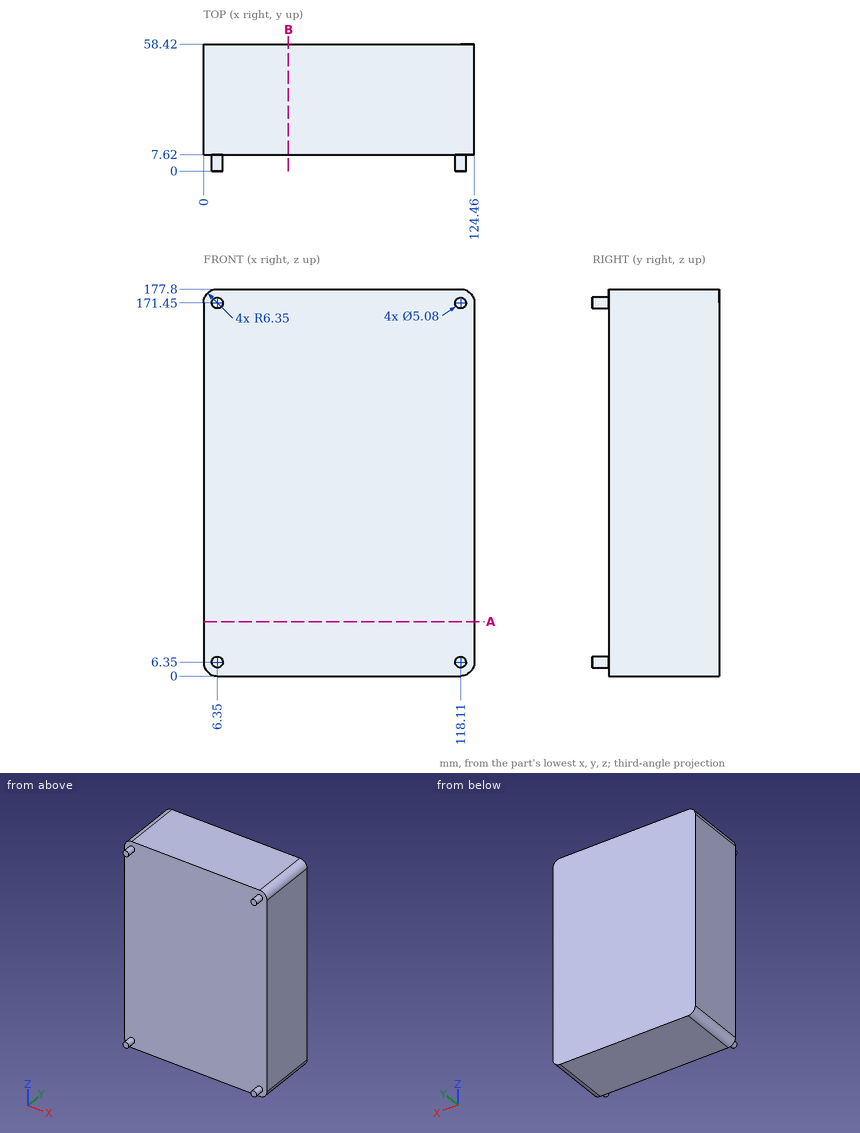
Geometry check sheet. Reference: drawing and pictorial views, mm from the part's lowest x, y, z. Give positions to 0.01 mm unless a question says otherwise; leave off trailing zeros. Order: outer loops, then holes, each group sorted by start corner. A loop starts at its lowest first (then second) coordinate and runs counter-clockwise, first axis right, second up. Notation, with made-up numbers: (81, -17.5) -> (98, -17.5) arc R15 ccw to (98, 4.5) -> close; hole circle Ø5 at (-4.5, -31). An arc over 180 degrees is marked (long way). Use CSV: the item, a comma, the result in double quotes. Start each with the question number.
1) Go/stop test with a flat-tipped pin: P1, Ø10, axis at x = 89, z = 45, coming from the -Y side. Record where the tip stops, or that it passes through.
2) Sectioned sample at A-A, the plane z = 25. Record the boundary of the cut face in (x, y), plus the area to 3 significant figures.
3) Sectioned sample at B-B, the plane x = 39. Record the boundary of the cut face in (y, z).
4) Material ranges on line 1 (Y direction, x = 61.5, z = 147.5), recorded low to high. Write a range as from..to.
Recorded:
1,P1,"y = 7.62"
2,outline,"(0, 7.62) -> (124.46, 7.62) -> (124.46, 58.42) -> (0, 58.42) -> close"
2,area,"6,320 mm2"
3,outline,"(7.62, 0) -> (58.42, 0) -> (58.42, 177.8) -> (7.62, 177.8) -> close"
4,line 1,"7.62..58.42"
